Input: part model. Units: mm. Frame: model coordinates. Face numbers are marked on the shaded views. A direction names the side the tool comes from. Round coordinates to 2 decimals unless told otherwise and drop trailing zeros. Order: outer loops, then holes, each group sorted by start corner. A loop starts at its lowest first (then second) coordinate and runs counter-clockwise, first axis right, second up. Notation, with made-up numbers: (-33.75, 71) -> (23.25, 71) arc R7 ccw to (23.25, 84) -> close; hole circle Ø5 at (63.25, 4.25). An arc over 180 degrees is marked (long way). Use a Markdown table: item, result.
from build123d import *

# Parameters (mm, degrees)
SKETCH1_W           = 152.4
SKETCH1_H           = 101.6
BOSS_EXTRUDE1_DEPTH = 25.4
SHELL1_T            = -0.8128
SKETCH3_W           = 171.45
SKETCH3_H           = 120.65
SKETCH3_W_2         = 152.4
SKETCH3_H_2         = 101.6
BOSS_EXTRUDE2_DEPTH = 0.8128


with BuildPart() as part:
    # Sketch1 → Boss-Extrude1 (new body)
    with BuildSketch(Plane(origin=(0, 0, 0), x_dir=(1, 0, 0), z_dir=(0, 1, 0))):
        Rectangle(SKETCH1_W, SKETCH1_H)
    extrude(amount=-BOSS_EXTRUDE1_DEPTH)

    # Shell1
    shell1_openings = [part.faces().sort_by_distance(p)[0] for p in [
        (0, 0, 0),
    ]]
    offset(amount=SHELL1_T, openings=shell1_openings, kind=Kind.INTERSECTION)

    # Sketch3 → Boss-Extrude2 (add)
    with BuildSketch(Plane(origin=(0, 0, 0), x_dir=(1, 0, 0), z_dir=(0, 1, 0))):
        Rectangle(SKETCH3_W, SKETCH3_H)
        Rectangle(SKETCH3_W_2, SKETCH3_H_2, mode=Mode.SUBTRACT)
    extrude(amount=-BOSS_EXTRUDE2_DEPTH)


solid = part.part
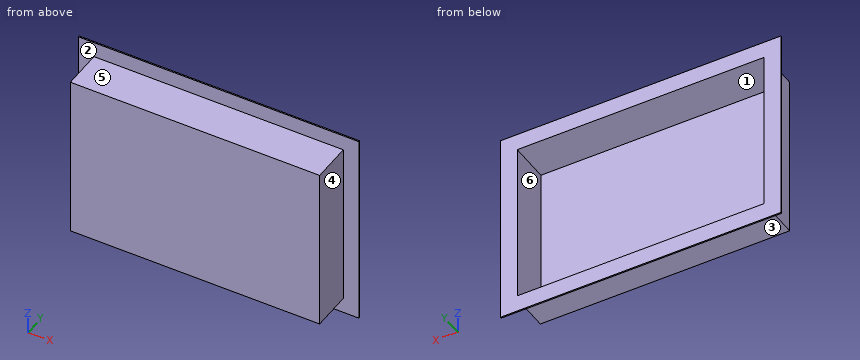
1) Cut plane B-B on z = -31. Return loops of the section in (x, y) (3 decimals).
Results found:
| item | result |
|---|---|
| outline | (-85.725, -0.813) -> (-76.2, -0.813) -> (-76.2, -25.4) -> (76.2, -25.4) -> (76.2, -0.813) -> (85.725, -0.813) -> (85.725, 0) -> (75.387, 0) -> (75.387, -24.587) -> (-75.387, -24.587) -> (-75.387, 0) -> (-85.725, 0) -> close |
2) Cut plane A-A on y = -21. Return loops of the section in (x, z).
Results found:
| item | result |
|---|---|
| outline | (-76.2, -50.8) -> (76.2, -50.8) -> (76.2, 50.8) -> (-76.2, 50.8) -> close; hole (-75.39, -49.99) -> (75.39, -49.99) -> (75.39, 49.99) -> (-75.39, 49.99) -> close |
3) Line query: L1, parallel to X at y = -23, z = 9; L2, parallel to Z at x = 9.5, y = -18.5; L3, parallel to Y at x = 26.5, z = -36.5. Output: solid intervals per line, ascending. Write a range as [from, to].
Results found:
| item | result |
|---|---|
| L1 | x = [-76.2, -75.39], [75.39, 76.2] |
| L2 | z = [-50.8, -49.99], [49.99, 50.8] |
| L3 | y = [-25.4, -24.59] |
4) Cut plane C-C on x = 26. Return loops of the section in (y, z) (3 decimals).
Results found:
| item | result |
|---|---|
| outline | (-25.4, -50.8) -> (-0.813, -50.8) -> (-0.813, -60.325) -> (0, -60.325) -> (0, -49.987) -> (-24.587, -49.987) -> (-24.587, 49.987) -> (0, 49.987) -> (0, 60.325) -> (-0.813, 60.325) -> (-0.813, 50.8) -> (-25.4, 50.8) -> close |
5) Set-up query: the marked faces 4, 5 and 6. Return all of +Z, -Z, +X, -X, +Y, -Y with unobstructed straight access to the full face (end or side cutting, diameter ignored); none if empty.
Results found:
| item | result |
|---|---|
| face 4 | +Z, -Z, +X, -Y |
| face 5 | +Z, +X, -X, -Y |
| face 6 | +Y |
6) Pull-direction query (Z, two-part tool) for the marked faces 1, 2 and 3; classes: +Z half, -Z half, draft (parallel to the pull), parting line (faces both ways), or undercut.
Results found:
| item | result |
|---|---|
| face 1 | undercut |
| face 2 | draft |
| face 3 | -Z half |
7) Pin query (flat end, axial travel): pin 1 Ø7.5 at (y, z) = (-12.5, -12.5) entering from -X; pin 2 Ø5 at (x, z) = (51, 6) entering from +Y; pin 3 Ø7.5 at (y, z) = (-7.5, -7.5) entering from +X. Return the tip coordinate at first contact, or that it passes through.
Results found:
| item | result |
|---|---|
| pin 1 | stops at x = -76.2 |
| pin 2 | stops at y = -24.59 |
| pin 3 | stops at x = 76.2 |
